Autodesk Inventor part; units mm, degrees
ref_plane "Work Plane1" through (0, 0, 10) normal (0, 0, 1) x (1, 0, 0)
ref_plane "YZ Plane" through (0, 0, 0) normal (1, 0, 0) x (0, 1, 0)
ref_plane "XZ Plane" through (0, 0, 0) normal (0, 1, 0) x (-1, 0, 0)
ref_plane "Work Plane1" through (0, 0, 10) normal (0, 0, 1) x (1, 0, 0)
sketch "Sketch1" plane through (0, 0, 10) normal (0, 0, 1) x (1, 0, 0)
  line L0 (-4.0299, -0.3538) -> (-2.2322, 1.4439) construction
  arc A0 (-1.4439, 2.2322) -> (-2.2322, 1.4439) centre (-0.9299, 0.9299) ccw construction
  line L1 (-1.4439, 2.2322) -> (0.3538, 4.0299) construction
  line L2 (-37.8299, 42.8299) -> (-37.8299, 37.8299) construction
  line L3 (-37.8299, 37.8299) -> (-42.9208, 37.8299) construction
  line L4 (-37.8299, 42.2137) -> (-37.8299, 45.8299) construction
  line L5 (-37.8299, 45.8299) -> (-4.0299, 45.8299) construction
  line L6 (-4.0299, 45.8299) -> (-4.0299, 42.2137) construction
  line L7 (-4.0299, 4.0299) -> (0.3538, 4.0299)
  circle A1 centre (-20.9299, 20.9299) radius 17.5
  line L8 (-20.9299, 58.9723) -> (17.1124, 20.9299) construction
  line L9 (17.1124, 20.9299) -> (-20.9299, -17.1124) construction
  line L10 (-20.9299, -17.1124) -> (-58.9723, 20.9299) construction
  line L11 (-58.9723, 20.9299) -> (-20.9299, 58.9723) construction
  line L12 (-20.9299, 58.9723) -> (-20.9299, -17.1124) construction
  line L13 (17.1124, 20.9299) -> (-58.9723, 20.9299) construction
  line L14 (-20.9299, 58.9723) -> (32.8701, 58.9723) construction
  line L15 (-43.4299, 43.4299) -> (1.5701, 43.4299) construction
  line L16 (1.5701, 43.4299) -> (1.5701, -1.5701) construction
  line L17 (1.5701, -1.5701) -> (-43.4299, -1.5701) construction
  line L18 (-43.4299, -1.5701) -> (-43.4299, 43.4299) construction
  line L19 (-43.4299, 43.4299) -> (1.5701, -1.5701) construction
  line L20 (1.5701, 43.4299) -> (-43.4299, -1.5701) construction
  line L21 (-43.4299, 5.3876) -> (-43.4299, 36.4723)
  line L22 (-43.4299, 36.4723) -> (-36.4723, 43.4299)
  line L23 (-36.4723, 43.4299) -> (-5.3876, 43.4299)
  line L24 (-5.3876, 43.4299) -> (1.5701, 36.4723)
  line L25 (1.5701, 36.4723) -> (1.5701, 5.3876)
  line L26 (1.5701, 5.3876) -> (-5.3876, -1.5701)
  line L27 (-5.3876, -1.5701) -> (-36.4723, -1.5701)
  line L28 (-36.4723, -1.5701) -> (-43.4299, 5.3876)
  line L29 (-4.0299, 42.2137) -> (-37.8299, 42.2137)
  line L30 (-4.0299, -0.3538) -> (-4.0299, 4.0299)
  circle A2 centre (-20.9299, 20.9299) radius 1.5
  line L31 (-10.9299, 10.9299) -> (-30.9299, 10.9299) construction
  line L32 (-30.9299, 10.9299) -> (-30.9299, 30.9299) construction
  line L33 (-30.9299, 30.9299) -> (-10.9299, 30.9299) construction
  line L34 (-10.9299, 30.9299) -> (-10.9299, 10.9299) construction
  line L35 (-10.9299, 10.9299) -> (-30.9299, 30.9299) construction
  line L36 (-30.9299, 10.9299) -> (-10.9299, 30.9299) construction
  circle A3 centre (-30.9299, 30.9299) radius 1.4
  circle A4 centre (-30.9299, 10.9299) radius 1.4
  circle A5 centre (-10.9299, 10.9299) radius 1.4
  line L37 (-45.8299, 37.8299) -> (-42.0723, 37.8299) construction
  line L38 (-42.1723, 37.7299) -> (-45.8299, 37.7299)
  line L39 (-45.8299, 37.7299) -> (-45.8299, 4.1299)
  line L40 (-45.8299, 4.1299) -> (-42.1723, 4.1299)
  line L41 (-42.1723, 4.1299) -> (-42.1723, 37.7299)
  line L42 (-45.8299, 4.0299) -> (-42.0723, 4.0299) construction
  line L43 (-45.8299, 37.8299) -> (-42.0723, 37.8299)
  line L44 (-37.7299, 45.8299) -> (-4.1299, 45.8299)
  line L45 (-4.1299, 45.8299) -> (-4.1299, 42.1723)
  line L46 (-4.1299, 42.1723) -> (-37.7299, 42.1723)
  line L47 (-37.7299, 42.1723) -> (-37.7299, 45.8299)
  line L48 (0.4701, 37.8299) -> (0.4701, 4.0299) construction
  line L49 (0.4701, 4.0299) -> (3.9701, 4.0299) construction
  line L50 (3.9701, 37.8299) -> (3.9701, 4.0299) construction
  line L51 (0.4701, 37.8299) -> (3.9701, 37.8299) construction
  line L52 (-45.8299, -3.9701) -> (-4.0299, -3.9701) construction
  line L53 (0.3124, 37.7299) -> (3.9701, 37.7299)
  line L54 (3.9701, 37.7299) -> (3.9701, 4.1299)
  line L55 (3.9701, 4.1299) -> (0.3124, 4.1299)
  line L56 (0.3124, 4.1299) -> (0.3124, 37.7299)
  line L57 (-4.1713, -0.3538) -> (-37.7299, -0.3538)
  line L58 (-37.7299, -0.3538) -> (-37.7299, -3.9701)
  line L59 (-37.7299, -3.9701) -> (-4.1713, -3.9701)
  line L60 (-4.1713, -3.9701) -> (-4.1713, -0.3538)
  point P0 (-37.8299, 4.0299)
  dimension "d18" = 53.8
  dimension "d19" = 45
  dimension "d20" = 53.8
  dimension "d21" = 45
  dimension "d22" = 45
  dimension "d30" = 20
  dimension "d31" = 20
  dimension "d32" = 2.8
  dimension "d33" = 2.8
  dimension "d34" = 2.8
  dimension "d35" = 3
  dimension "d36" = 0.1
  dimension "d37" = 0.1
  dimension "d38" = 0.1
  dimension "d39" = 0.1
extrude "Extrusion1" add sketch "Sketch1" along normal blind 8 contours L30 L26 L57 L28 L41 L22 L46 L24 L56 L7 | L7 L26 L30 | L56 L24 L25 L26 | L26 L25 L24 L53 L54 L55 | L60 L59 L58 L57 L28 L27 L26 | L26 L27 L28 L57 | L46 L22 L29 L24 | L24 L29 L45 | L40 L39 L38 L22 L21 L28 | L28 L21 L22 L41 | L29 L22 L23 L24 | L24 L23 L22 L29 L47 L44 L45 | L47 L29 L22 | A1 | A2 | A3 | A4 | A5
sketch "Skizze4" plane through (0, 0, 18) normal (0, 0, 1) x (1, 0, 0)
  line L0 (-37.7299, 42.1723) -> (-42.1723, 37.7299)
  line L1 (-42.1723, 37.7299) -> (-45.8299, 37.7299)
  line L2 (-45.8299, 37.7299) -> (-45.8299, 4.1299) construction
  line L3 (-45.8299, 4.1299) -> (-42.1723, 4.1299)
  line L4 (-42.1723, 4.1299) -> (-37.6885, -0.3538)
  line L5 (-37.6885, -0.3538) -> (-37.7299, -0.3538)
  line L6 (-37.7299, -0.3538) -> (-37.7299, -3.9701)
  line L7 (-37.7299, -3.9701) -> (-4.1713, -3.9701) construction
  line L8 (-4.1713, -3.9701) -> (-4.1713, -0.3538)
  line L9 (-4.1713, -0.3538) -> (0.3124, 4.1299)
  line L10 (0.3124, 4.1299) -> (3.9701, 4.1299)
  line L11 (3.9701, 4.1299) -> (3.9701, 37.7299) construction
  line L12 (3.9701, 37.7299) -> (0.3124, 37.7299)
  line L13 (0.3124, 37.7299) -> (-4.1299, 42.1723)
  line L14 (-4.1299, 42.1723) -> (-4.1299, 45.8299)
  line L15 (-4.1299, 45.8299) -> (-37.7299, 45.8299) construction
  line L16 (-37.7299, 45.8299) -> (-37.7299, 42.1723)
  line L17 (-37.9299, 46.0299) -> (-3.9299, 46.0299) construction
  line L18 (-3.9299, 46.0299) -> (-3.9299, 42.2551)
  line L19 (-3.9299, 42.2551) -> (0.3953, 37.9299)
  line L20 (0.3953, 37.9299) -> (4.1701, 37.9299)
  line L21 (4.1701, 37.9299) -> (4.1701, 3.9299) construction
  line L22 (4.1701, 3.9299) -> (0.3953, 3.9299)
  line L23 (0.3953, 3.9299) -> (-3.9713, -0.4367)
  line L24 (-3.9713, -0.4367) -> (-3.9713, -4.1701)
  line L25 (-3.9713, -4.1701) -> (-37.9299, -4.1701) construction
  line L26 (-37.9299, -4.1701) -> (-37.9299, -0.3953)
  line L27 (-37.9299, -0.3953) -> (-42.2551, 3.9299)
  line L28 (-42.2551, 3.9299) -> (-46.0299, 3.9299)
  line L29 (-46.0299, 3.9299) -> (-46.0299, 37.9299) construction
  line L30 (-46.0299, 37.9299) -> (-42.2551, 37.9299)
  line L31 (-42.2551, 37.9299) -> (-37.9299, 42.2551)
  line L32 (-37.9299, 42.2551) -> (-37.9299, 46.0299)
  line L33 (-45.8299, 37.7299) -> (-45.8299, 37.9299)
  line L34 (-4.1299, 45.8299) -> (-37.7299, 45.8299)
  line L35 (-37.7299, 45.8299) -> (-37.9299, 45.8299)
  line L36 (-4.1299, 45.8299) -> (-3.9299, 45.8299)
  line L37 (3.9701, 37.7299) -> (3.9701, 37.9299)
  line L38 (3.9701, 4.1299) -> (3.9701, 37.7299)
  line L39 (3.9701, 4.1299) -> (3.9701, 3.9299)
  line L40 (-4.1713, -3.9701) -> (-3.9713, -3.9701)
  line L41 (-37.7299, -3.9701) -> (-37.9299, -3.9701)
  line L42 (-45.8299, 4.1299) -> (-45.8299, 3.9299)
  point P0 (0, 0)
  dimension "d40" = 0.2
extrude "IM_offset" add sketch "Skizze4" against normal up to surface (8 mm away)
ref_plane "Arbeitsebene5" through (-20.9299, 3.9299, 10) normal (1, 0, 0) x (0, 0, -1)
ref_plane "Arbeitsebene6" through (-37.9299, 20.9299, 10) normal (0, 1, 0) x (1, 0, 0)
sketch "Skizze25" plane through (0, 0, 10) normal (0, 0, -1) x (-1, 0, 0)
  line L0 (3.9713, -3.9701) -> (37.9299, -3.9701)
  line L1 (37.9299, -3.9701) -> (37.9299, -0.3953)
  line L2 (37.9299, -0.3953) -> (42.2551, 3.9299)
  line L3 (42.2551, 3.9299) -> (45.8299, 3.9299)
  line L4 (45.8299, 3.9299) -> (45.8299, 37.9299)
  line L5 (45.8299, 37.9299) -> (42.2551, 37.9299)
  line L6 (42.2551, 37.9299) -> (37.9299, 42.2551)
  line L7 (37.9299, 42.2551) -> (37.9299, 45.8299)
  line L8 (37.9299, 45.8299) -> (3.9299, 45.8299)
  line L9 (3.9299, 45.8299) -> (3.9299, 42.2551)
  line L10 (3.9299, 42.2551) -> (-0.3953, 37.9299)
  line L11 (-0.3953, 37.9299) -> (-3.9701, 37.9299)
  line L12 (-3.9701, 37.9299) -> (-3.9701, 3.9299)
  line L13 (-3.9701, 3.9299) -> (-0.3953, 3.9299)
  line L14 (-0.3953, 3.9299) -> (3.9713, -0.4367)
  line L15 (3.9713, -0.4367) -> (3.9713, -3.9701)
  circle A0 centre (20.9299, 32.9299) radius 4
  circle A1 centre (20.9299, 8.9299) radius 4
  line L16 (-13.9301, 20.9299) -> (55.7899, 20.9299)
  line L17 (10.9299, 13.4299) -> (30.9299, 13.4299)
  line L18 (30.9299, 13.4299) -> (30.9299, 28.4299)
  line L19 (30.9299, 28.4299) -> (10.9299, 28.4299)
  line L20 (10.9299, 28.4299) -> (10.9299, 13.4299)
  line L21 (10.9299, 13.4299) -> (30.9299, 28.4299) construction
  line L22 (30.9299, 13.4299) -> (10.9299, 28.4299) construction
  point P0 (0, 0)
  point P1 (20.9299, 20.9299)
  dimension "d150" = 8
  dimension "d151" = 8
  dimension "d152" = 12
  dimension "d153" = 12
  dimension "d154" = 20
  dimension "d155" = 15
hole "Bohrung1" at (-30.9299, 28.4299, 10) at (-30.9299, 13.4299, 10) at (-10.9299, 13.4299, 10) at (-10.9299, 28.4299, 10) direction (0, 0, 1) diameter 8 end through all
sketch "Skizze26" plane through (0, 0, 10) normal (0, 0, -1) x (-1, 0, 0)
  circle A0 centre (10.9299, 13.4299) radius 4
  circle A1 centre (30.9299, 28.4299) radius 4
  circle A2 centre (30.9299, 13.4299) radius 4
  circle A3 centre (10.9299, 28.4299) radius 4
  line L0 (3.9713, -3.9701) -> (37.9299, -3.9701)
  line L1 (37.9299, -3.9701) -> (37.9299, -0.3953)
  line L2 (37.9299, -0.3953) -> (42.2551, 3.9299)
  line L3 (42.2551, 3.9299) -> (45.8299, 3.9299)
  line L4 (45.8299, 3.9299) -> (45.8299, 37.9299)
  line L5 (45.8299, 37.9299) -> (42.2551, 37.9299)
  line L6 (42.2551, 37.9299) -> (37.9299, 42.2551)
  line L7 (37.9299, 42.2551) -> (37.9299, 45.8299)
  line L8 (37.9299, 45.8299) -> (3.9299, 45.8299)
  line L9 (3.9299, 45.8299) -> (3.9299, 42.2551)
  line L10 (3.9299, 42.2551) -> (-0.3953, 37.9299)
  line L11 (-0.3953, 37.9299) -> (-3.9701, 37.9299)
  line L12 (-3.9701, 37.9299) -> (-3.9701, 3.9299)
  line L13 (-3.9701, 3.9299) -> (-0.3953, 3.9299)
  line L14 (-0.3953, 3.9299) -> (3.9713, -0.4367)
  line L15 (3.9713, -0.4367) -> (3.9713, -3.9701)
  line L16 (8.7057, 18.1542) -> (33.7057, 18.1542)
  line L17 (33.7057, 18.1542) -> (33.7057, 23.1542)
  line L18 (33.7057, 23.1542) -> (8.7057, 23.1542)
  line L19 (8.7057, 23.1542) -> (8.7057, 18.1542)
  line L20 (8.7057, 18.1542) -> (33.7057, 23.1542) construction
  line L21 (33.7057, 18.1542) -> (8.7057, 23.1542) construction
  point P0 (0, 0)
  point P1 (21.2057, 20.6542)
  dimension "d163" = 25
  dimension "d164" = 5
extrude "Extrusion21" cut sketch "Skizze26" against normal blind 10 contours L19 L18 L17 L16
properties part number "20_Cube_Insert_Filter_25mm"
For this review, take the finished solid that the model builds, in its own axes (mm). A direction names the side the tool comes from. Round coordinates to 2 decimals unless told otherwise and drop trailing zeros. Loops run counter-clockwise (first coordinate to the right, second up) from the corner with the lowest first, then second, coordinate; pieces in that order, holes last.
(1) Mouldability with a two-part tool opening along X and no side actions: class faces 1 (the flat face through (-1.798, 40.123, 14.056)), 2 (the flat face through (-37.93, 44, 14)), 3 (the cylindrical face through (-14.896, 12.909, 14.056)) as released by +X, released by -X, zero draft, split by the parting line, or undercut.
Returned:
face 1: released by +X
face 2: released by -X
face 3: undercut
(2) Tool access review of faces 4 (the flat face through (-21, 23.154, 14)), 5 (the flat face through (2, 3.93, 14)), 6 (the flat face through (-37.93, -2, 14)), 7 (the flat face through (-3.93, 44, 14)): name each direction out of +Z, -Z, +X, -X, +Y, -Y from which nothing blocks a thin tool from reaching the whole face with its end or side.
Returned:
face 4: +Z, -Z
face 5: +Z, -Z, +X, -Y
face 6: +Z, -Z, -X, -Y
face 7: +Z, -Z, +X, +Y
(3) We need section D-D (y = 20). Give the boundary of the cut face in (x, z).
Returned:
outline: (-45.83, 10) - (-33.71, 10) - (-33.71, 18) - (-45.83, 18) - close; (-8.71, 10) - (3.97, 10) - (3.97, 18) - (-8.71, 18) - close
(4) Clearance check with flat-ended pins moving along their axes: P1, Ø1.8, axis at y = -3, z = 14, coming from the +X side; P2, Ø1.8, axis at y = -1.5, z = 15.5, coming from the -X side; P3, Ø3, axis at x = -44.5, z = 14, coming from the -Y side. State where each tip first meets the part, or that it passes through.
Returned:
P1: stops at x = -3.97
P2: stops at x = -37.93
P3: stops at y = 3.93
(5) Wall thickness on line 1 along X through (y, z) = (28.5, 12.75); line 2 along Y through (x, z) = (-21, 11); line 3 along X through (y, z) = (21, 14): over which ranges is each line inside the solid? List them lowest first.
Returned:
line 1: x = -45.83 to -34.93, -26.93 to -14.93, -6.93 to 3.97
line 2: y = -3.97 to 18.15, 23.15 to 45.83
line 3: x = -45.83 to -33.71, -8.71 to 3.97
(6) We need section B-B (y = 30). Give the boundary of the cut face in (x, z).
Returned:
outline: (-45.83, 10) - (-34.61, 10) - (-34.61, 18) - (-45.83, 18) - close; (-27.25, 10) - (-14.61, 10) - (-14.61, 18) - (-27.25, 18) - close; (-7.25, 10) - (3.97, 10) - (3.97, 18) - (-7.25, 18) - close
(7) We need section A-A (x = -18.5). Give the boundary of the cut face in (y, z), plus the area to 3 significant figures.
Returned:
outline: (-3.97, 10) - (18.15, 10) - (18.15, 18) - (-3.97, 18) - close; (23.15, 10) - (45.83, 10) - (45.83, 18) - (23.15, 18) - close
area: 358 mm2
(8) We need section C-C (x = -27.5). Give the boundary of the cut face in (y, z), plus the area to 3 significant figures.
Returned:
outline: (-3.97, 10) - (11.37, 10) - (11.37, 18) - (-3.97, 18) - close; (15.49, 10) - (18.15, 10) - (18.15, 18) - (15.49, 18) - close; (23.15, 10) - (26.37, 10) - (26.37, 18) - (23.15, 18) - close; (30.49, 10) - (45.83, 10) - (45.83, 18) - (30.49, 18) - close
area: 293 mm2
